Design review of the part shown in the three views and the two pictorial views. Dimensions are in mm from the part's minimum x, y and z. Give positions to 0.01 mm unless a question says otherwise; leave off trailing zeros. Write each loop counter-clockwise with the first axis right and the second up, starting at its lowest first coordinate (ties: lowest second). Pieces come first, ordered by that corner, then holes. Notation, with made-up numbers: M 11.25,7.5 L 44.25,7.5 A26 cw 44.25,23.5 Z; hole C 9.5,8 d11. An arc over 180 degrees is marked long. Use one line per item in the form item = value. Start each with the question number.
Q1. Clearance check with flat-ended pins moving along their axes: pin 1 Ø3 at (x, y) = (136.25, 111) entering from -Z; pin 2 Ø1.5 at (x, y) = (15, 55.5) entering from -Z. State where each tip first meets the part, or that it passes through.
Q2. Consider section B-B on y = 31. Write out the cut boundary in (x, z).
Q3. Consider section C-C on z = 4.2. Give the number of separate pieces and of enclosed holes in the cut face, and give its area (3 significant figures).
Q4. Consider section A-A on x = 136.25. Write out the cut boundary in (y, z).
Q5. For probe 1 along X at (y, z) = (137, 3.85); probe 2 along Y at (x, z) = (36.25, 1.75); probe 3 along Y at (x, z) = (108, 4), list the stretches that pass through material, from the lowest coordinate up. Write a range as [from, to].
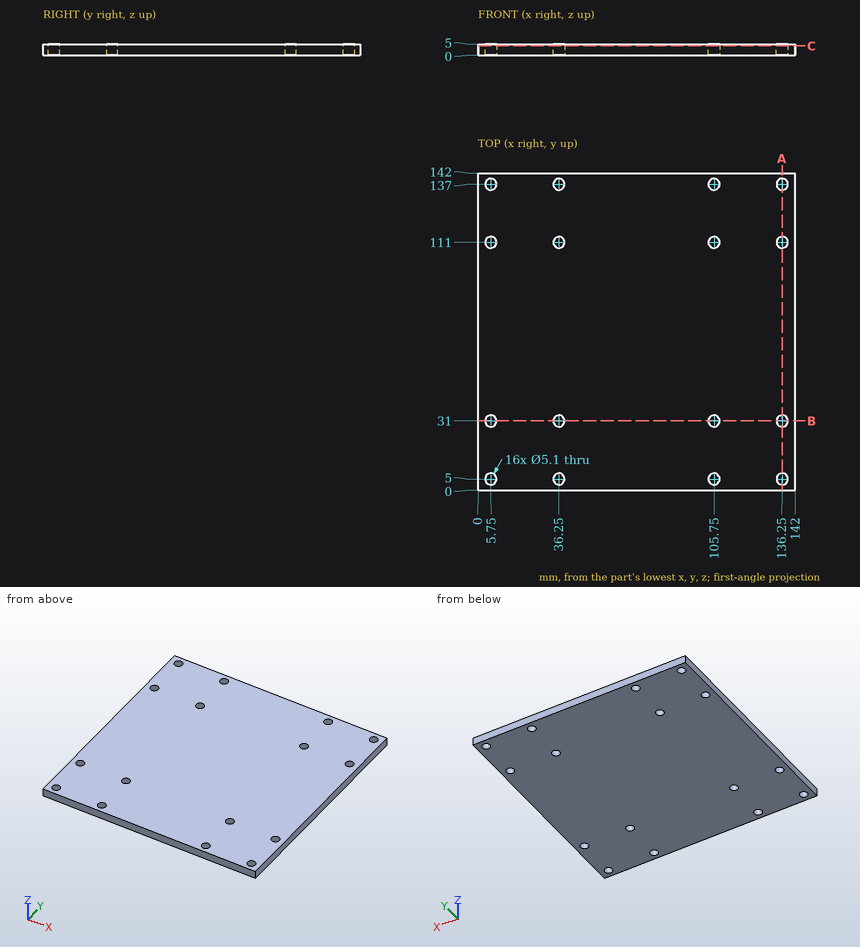
Working result:
q1.pin_1 = through
q1.pin_2 = 0
q2.outline = M 0,0 L 3.2,0 L 3.2,5 L 0,5 Z; M 8.3,0 L 33.7,0 L 33.7,5 L 8.3,5 Z; M 38.8,0 L 103.2,0 L 103.2,5 L 38.8,5 Z; M 108.3,0 L 133.7,0 L 133.7,5 L 108.3,5 Z; M 138.8,0 L 142,0 L 142,5 L 138.8,5 Z
q3.separate_pieces = 1
q3.enclosed_holes = 16
q3.area = 19,800 mm²
q4.outline = M 0,0 L 2.45,0 L 2.45,5 L 0,5 Z; M 7.55,0 L 28.45,0 L 28.45,5 L 7.55,5 Z; M 33.55,0 L 108.45,0 L 108.45,5 L 33.55,5 Z; M 113.55,0 L 134.45,0 L 134.45,5 L 113.55,5 Z; M 139.55,0 L 142,0 L 142,5 L 139.55,5 Z
q5.probe_1 = [0, 3.2], [8.3, 33.7], [38.8, 103.2], [108.3, 133.7], [138.8, 142]
q5.probe_2 = [0, 2.45], [7.55, 28.45], [33.55, 108.45], [113.55, 134.45], [139.55, 142]
q5.probe_3 = [0, 3.8], [6.2, 29.8], [32.2, 109.8], [112.2, 135.8], [138.2, 142]
